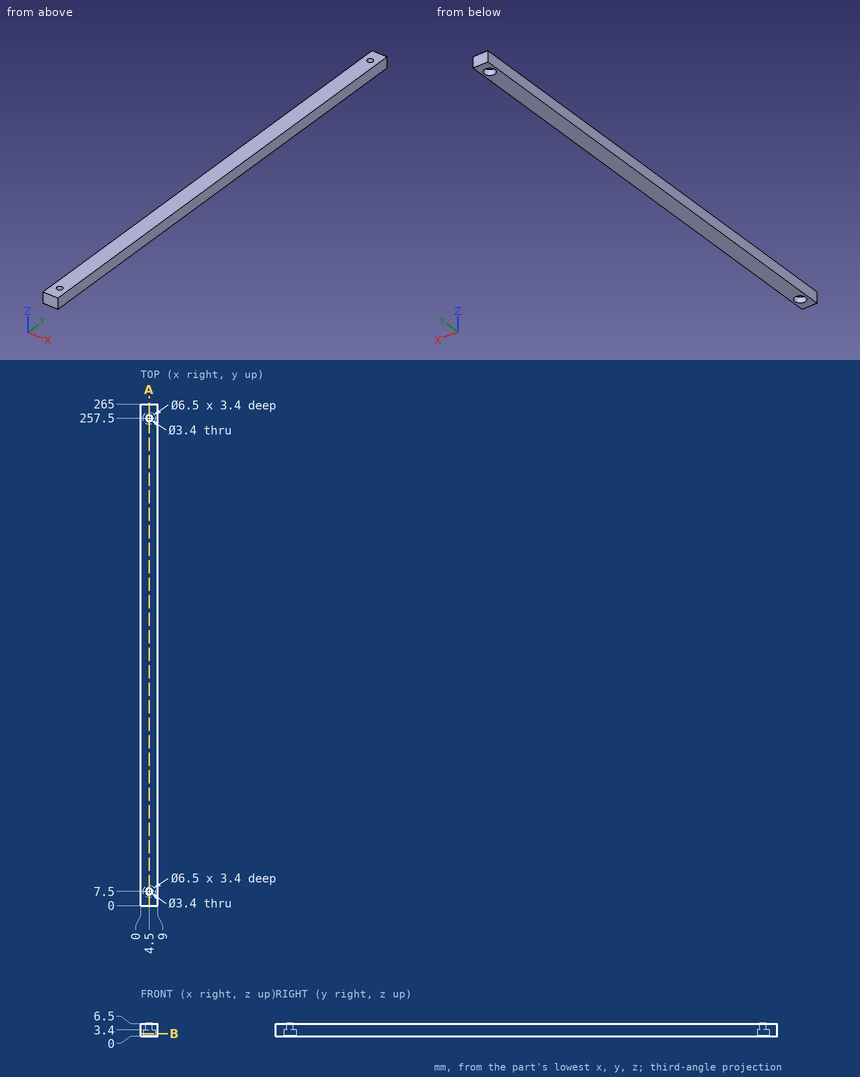
Design review of the part shown in the three views and the two pictorial views. Dimensions are in mm from the part's minimum x, y and z. Give positions to 0.01 mm unless a question says otherwise; leave off trailing zeros. Loops run counter-clockwise (first coordinate to the right, second up) from the corner with the lowest first, then second, coordinate; pieces in that order, holes last. Notation, with made-up numbers: (23.5, -30.5) - (28.5, -30.5) arc R15 cw to (28.5, -4.5) - close; hole circle Ø11 at (70, 57). An arc over 180 degrees is marked (long way). Write item = value, one per line.
1) Take a section at A-A on x = 4.5. State the section outline as (y, z) points, and give its area (3 significant figures).
Result sheet:
outline = (0, 0) - (4.25, 0) - (4.25, 3.4) - (5.8, 3.4) - (5.8, 6.5) - (0, 6.5) - close; (9.2, 3.4) - (10.75, 3.4) - (10.75, 0) - (254.25, 0) - (254.25, 3.4) - (255.8, 3.4) - (255.8, 6.5) - (9.2, 6.5) - close; (259.2, 3.4) - (260.75, 3.4) - (260.75, 0) - (265, 0) - (265, 6.5) - (259.2, 6.5) - close
area = 1,660 mm2
2) Take a section at B-B on z = 1.25. State the section outline as (x, y) points.
Result sheet:
outline = (0, 0) - (9, 0) - (9, 265) - (0, 265) - close; hole circle Ø6.5 at (4.5, 7.5); hole circle Ø6.5 at (4.5, 257.5)
3) To check wall thickness, follow line 1 (Y direction, x = 6.25, z = 0.75); line 2 (Y direction, x = 4.5, z = 5.55); line 3 (X direction, y = 257.5, z = 0.75). State the ranges of each line that lie inside material, in increasing order.
Result sheet:
line_1 = 0 to 4.76, 10.24 to 254.76, 260.24 to 265
line_2 = 0 to 5.8, 9.2 to 255.8, 259.2 to 265
line_3 = 0 to 1.25, 7.75 to 9
4) Clearance check with a flat-ended pin moving along its axis: pin 1 Ø2 at (x, y) = (4, 9) entering from -Z. State where the tip first meets the part, or that it passes through.
Result sheet:
pin_1 = 3.4
